Source: CAD feature listing. Evaluate the final solid. Frame: model axes, mm. A direction names the side the tool comes from. Give positions to 0.01 mm unless a question says otherwise; leave off trailing zeros. Loops run counter-clockwise (first coordinate to the right, second up) from the corner with the lowest first, then second, coordinate; pieces in that order, holes last. Notation, with made-up numbers: (-15.75, -28) -> (11.25, -28) arc R24 ccw to (11.25, -16) -> close; hole circle Ø4 at (86.25, 87). An arc over 180 degrees is marked (long way). Answer as a JSON object with one key per item and string values. Group by question number.
Autodesk Inventor part; units mm, degrees
ref_plane "Work Plane1" through (0, 0, -26.75) normal (0, 0, -1) x (-1, 0, 0)
ref_plane "Work Plane2" through (18, 0, 0) normal (1, 0, 0) x (0, 1, 0)
ref_plane "Work Plane3" through (0, 0, 26.5) normal (0, 0, -1) x (-1, 0, 0)
sketch "Sketch1" plane through (0, 0, 0) normal (0, 0, 1) x (1, 0, 0)
  circle A0 centre (0, 0) radius 17.75
  dimension "d0" = 35.5
extrude "Extrusion1" add sketch "Sketch1" along normal mid plane 57
fillet "Fillet1" radius 2 1 edges at (-17.75, 0, 28.5)
shell "Shell1" thickness 0.62 removed faces 1 at (3.0438, 4.2648, -28.5)
sketch "Sketch2" plane through (0, 0, 28.5) normal (0, 0, 1) x (1, 0, 0)
  circle A0 centre (0, 0) radius 15.75
  circle A1 centre (0, 0) radius 6.5
  dimension "d5" = 13
extrude "Extrusion2" add sketch "Sketch2" along normal blind 4.5 contours A1
fillet "Fillet2" radius 0.5 2 edges at (-6.5, 0, 28.5) (-6.5, 0, 33)
sketch "Sketch3" plane through (0, 0, 33) normal (0, 0, 1) x (1, 0, 0)
  circle A0 centre (0, 0) radius 6
  circle A1 centre (0, 0) radius 1.6
  dimension "d9" = 3.2
extrude "Extrusion3" add sketch "Sketch3" along normal blind 10 contours A1
fillet "Fillet3" radius 1.6 1 edges at (-1.6, 0, 43)
sketch "Sketch4" plane through (0, 0, 28.5) normal (0, 0, 1) x (1, 0, 0)
  circle A0 centre (0, 0) radius 15.75
  point P0 (12.5, 0)
  dimension "d13" = 12.5
hole "Hole1" at (12.5, 0, 28.5) direction (0, 0, -1) diameter 2.5 depth 8 tip angle 118
mirror "Mirror1" about plane through (0, 0, 0) normal (1, 0, 0) of "Hole1"
sketch "Sketch5" plane through (0, 0, 28.5) normal (0, 0, 1) x (1, 0, 0)
  circle A0 centre (12.5, 0) radius 1.25
  circle A1 centre (0, 0) radius 7
  arc A2 (12.557, 3.3646) -> (3.3646, 12.557) centre (0, 0) ccw
  arc A3 (9.1763, 2.4588) -> (2.4588, 9.1763) centre (0, 0) ccw
  line L0 (0, 0) -> (3.3646, 12.557) construction
  line L1 (0, 0) -> (12.557, 3.3646) construction
  line L2 (2.4588, 9.1763) -> (3.3646, 12.557)
  line L3 (9.1763, 2.4588) -> (12.557, 3.3646)
  line L4 (0, 0) -> (12.5, 0) construction
  line L5 (0.151, 0.5634) -> (0.151, 14.7153) construction
  dimension "d21" = 15
  dimension "d22" = 15
  dimension "d23" = 13
  dimension "d24" = 9.5
extrude "Extrusion4" cut sketch "Sketch5" against normal blind 10 contours L3 A3 L2 A2
pattern_circular "Circular Pattern1" count 4 over 360 about axis through (0, 0, 0) along (0, 0, 1) of "Extrusion4"
ref_plane "Work Plane1" through (0, 0, -26.75) normal (0, 0, -1) x (-1, 0, 0)
sketch "Sketch6" plane through (0, 0, -26.75) normal (0, 0, -1) x (-1, 0, 0)
  circle A0 centre (0, 0) radius 17.13
extrude "Extrusion5" add sketch "Sketch6" against normal blind 0.62
sketch "Sketch7" plane through (0, 0, -26.75) normal (0, 0, -1) x (-1, 0, 0)
  circle A0 centre (0, 0) radius 17.13
  circle A1 centre (0, 0) radius 12
  dimension "d33" = 24
extrude "Extrusion6" add sketch "Sketch7" along normal blind 0.62 contours A1
sketch "Sketch8" plane through (0, 0, -27.37) normal (0, 0, -1) x (-1, 0, 0)
  circle A0 centre (0, 0) radius 12
  circle A1 centre (0, 0) radius 5.375
  dimension "d36" = 10.75
extrude "Extrusion7" add sketch "Sketch8" along normal blind 3 contours A1
sketch "Sketch9" plane through (0, 0, -30.37) normal (0, 0, -1) x (-1, 0, 0)
  circle A0 centre (0, 0) radius 5.375
  circle A1 centre (0, 0) radius 3.45
  dimension "d39" = 6.9
extrude "Extrusion8" cut sketch "Sketch9" against normal blind 0.8 contours A1
sketch "Sketch10" plane through (0, 0, -29.57) normal (0, 0, -1) x (-1, 0, 0)
  circle A0 centre (0, 0) radius 3.45
  circle A1 centre (0, 0) radius 1.6
  dimension "d42" = 3.2
extrude "Extrusion9" add sketch "Sketch10" along normal blind 1 contours A1
sketch "Sketch11" plane through (0, 0, -27.37) normal (0, 0, -1) x (-1, 0, 0)
  circle A0 centre (0, 0) radius 5.375
  circle A1 centre (0, 0) radius 12
  arc A2 (9.3591, 3.15) -> (3.15, 9.3591) centre (0, 0) ccw
  arc A3 (5.6857, 3.15) -> (3.15, 5.6857) centre (0, 0) ccw
  line L0 (3.15, 9.3591) -> (3.15, 5.6857)
  line L1 (5.6857, 3.15) -> (9.3591, 3.15)
  dimension "d45" = 3.15
  dimension "d46" = 3.15
  dimension "d47" = 9.875
  dimension "d48" = 6.5
extrude "Extrusion10" cut sketch "Sketch11" against normal blind 1 contours L1 A3 L0 A2
pattern_circular "Circular Pattern2" count 4 over 360 about axis through (0, 0, 0) along (0, 0, 1) of "Extrusion10"
sketch "Sketch12" plane through (0, 0, -26.75) normal (0, 0, -1) x (-1, 0, 0)
  circle A0 centre (0, 0) radius 12
  circle A1 centre (0, 0) radius 17.13
  line L0 (-14.5, 1.9) -> (-14, 1.9)
  line L1 (-14, 1.9) -> (-14, -1.9)
  line L2 (-14, -1.9) -> (-14.5, -1.9)
  line L3 (-14.5, -1.9) -> (-14.5, 1.9)
  line L4 (0, 0) -> (-16.9017, 0) construction
  point P0 (-14, 0)
  dimension "d54" = 0.5
  dimension "d55" = 3.8
  dimension "d56" = 14
extrude "Extrusion11" add sketch "Sketch12" along normal blind 7.2 contours L0 L1 L2 L3
chamfer "Chamfer1" distance 1 angle 45 2 edges at (14.25, 1.9, -33.95) (14.25, -1.9, -33.95)
sketch "Sketch13" plane through (14.5, -1.9, -26.75) normal (1, 0, 0) x (0, 0, -1)
  line L0 (7.2, 1) -> (7.2, 2.8)
  line L1 (4.2, 1.9) -> (6.2, 3.8) construction
  line L2 (4.2, 1.9) -> (6.2, 0) construction
  dimension "d61" = 3
hole "Hole2" at (14.5, 0, -30.95) direction (-1, 0, 0) diameter 2 depth 1 tip angle 118
mirror "Mirror2" about plane through (0, 0, 0) normal (1, 0, 0) of "Extrusion11", "Chamfer1", "Hole2"
ref_plane "Work Plane2" through (18, 0, 0) normal (1, 0, 0) x (0, 1, 0)
sketch "Sketch14" plane through (18, 0, 0) normal (1, 0, 0) x (0, 1, 0)
  arc A0 (-4.5554, -11.85) -> (-4.5554, -17.75) centre (-4.5554, -14.8) ccw
  arc A1 (5.2946, -17.75) -> (5.2946, -11.85) centre (5.2946, -14.8) ccw
  line L0 (-4.5554, -11.85) -> (5.2946, -11.85)
  line L1 (-4.5554, -17.75) -> (5.2946, -17.75)
  line L2 (17.75, -28.5) -> (-17.75, -28.5)
  line L3 (0, -28.5) -> (0, 17.1564) construction
  dimension "d70" = 10.75
  dimension "d71" = 5.9
  dimension "d72" = 9.85
extrude "Extrusion12" cut sketch "Sketch14" against normal through all
ref_plane "Work Plane3" through (0, 0, 26.5) normal (0, 0, -1) x (-1, 0, 0)
sketch "Sketch15" plane through (0, 0, 26.5) normal (0, 0, -1) x (-1, 0, 0)
  circle A0 centre (0, 0) radius 17.75
  circle A1 centre (0, 0) radius 19.25
  dimension "d76" = 1.5
extrude "Flux Ring" add sketch "Sketch15" along normal blind 38
properties part number "RS-550" material "Steel, Mild"
(1) Section query D-D on z = 35. Return the cut outline in (x, y), plus the area to 3 significant figures.
(2) Access query for faces 1 (the face through (-14.25, 0.04, -29.95)), 2 (the face through (-15.474, 8.245, -14.822)), 3 (the face through (6, 6, -26.37)). Directions: +Z, -Z, +X, -X, +Y, -Y. A direction counts if a zero-diameter tool reaches every point of the face in a straight line with its end or side. Return the directions, or none.
(3) First-contact query: pin 1 (1.1 mm diameter, centred on y = 0.5, z = -31, fed in from -X); pin 2 (0.8 mm diameter, centred on y = -8, z = -27, fed in from +X); pin 3 (10 mm diameter, centred on x = -10.5, z = -22, fed in from -Y); pin 4 (1.5 mm diameter, centred on x = -12, z = 29.5, fed in from +Y). Flat tips, straight axial feed; report the tip coordinate or a pass-through.
(4) Section query A-A on z = -14.8. Return the cut outline in (x, y).
(5) Section query C-C on z = 15.5. Return the cut outline in (x, y).
(6) Mould query, pull axis X, two halves, no side actions, for faces 4 (the face through (14.25, -0.04, -29.95)), 5 (the face through (-17.733, 0.78, -19.881)), 6 (the face through (-4, 12, -26.75)). Classes: pulls with the +X half, pulls with the -X half, needs draft (parallel to the pull), parting line crosses it, or undercut.
(7) Material intervals for line 1 (Z direction, x = -14.2, y = 0); line 2 (X direction, y = 0.5, z = 22); line 3 (Y direction, x = 0, z = -30) (3 decimals), sorted ascending. Write a range as from..to.
(8) Section query B-B on y = 0. State how many separate pieces and enclosed holes the cut face has, plus the area to 3 significant figures.
Result:
{
 "1": {"outline": "circle Ø3.2 at (0, 0)", "area": "8.04 mm²"},
 "2": {"face 1": "-X", "face 2": "+X, -X", "face 3": "-Z"},
 "3": {"pin 1": "x = -14.5", "pin 2": "x = 16.04", "pin 3": "y = -16.88", "pin 4": "through"},
 "4": {"outline": "(-16.09, -7.51) arc R17.75 ccw to (16.09, -7.51) -> (15.4, -7.51) arc R17.13 cw to (-15.4, -7.51) -> close; (-15.72, 8.24) -> (-15.02, 8.24) arc R17.13 cw to (15.02, 8.24) -> (15.72, 8.24) arc R17.75 ccw to start"},
 "5": {"outline": "circle Ø38.5 at (0, 0); hole circle Ø34.26 at (0, 0)"},
 "6": {"face 4": "needs draft", "face 5": "parting line crosses it", "face 6": "undercut"},
 "7": {"line 1": "-33.95..-31.95, -29.95..-26.13, 27.88..28.5", "line 2": "-19.24..-17.12, 17.12..19.24", "line 3": "-5.375..-3.45, -1.6..1.6, 3.45..5.375"},
 "8": {"separate pieces": "6", "enclosed holes": "0", "area": "355 mm²"}
}
